Geometry: final body of the model. Coordinates: model frame, mm. Face numbers are marked on the shaded views. A direction names the side the tool comes from. Give positions to 0.01 mm unless a question says otherwise; leave off trailing zeros. Order: outer loops, then holes, each group sorted by start corner. A loop starts at its lowest first (then second) coordinate and runs counter-clockwise, first axis right, second up. Notation, with made-up numbers: (31, 44.5) -> (81, 44.5) arc R32 ccw to (81, 72.5) -> close; hole circle Ø11 at (47.25, 27.5). An arc over 180 degrees is marked (long way). One line per item, written item: value. Start each with the question number.
```python
from build123d import *

# Parameters (mm, degrees)
F0_W     = 37
F0_H     = 37
F0_W_2   = 28
F0_H_2   = 30.4
F1_DEPTH = 4.5
F2_W     = 35
F2_H     = 33
F3_DEPTH = 2
F4_R     = 1.75
F5_DEPTH = 4
F6_DEPTH = 4
F7_R     = 1


with BuildPart() as f1:
    # F0 (on Top) → F1 (new body)
    with BuildSketch(Plane.XY):
        with Locations((-7.463294, -0.689729)):
            Rectangle(F0_W, F0_H)
        with Locations((-6.963294, -0.689729)):
            Rectangle(F0_W_2, F0_H_2, mode=Mode.SUBTRACT)
    extrude(amount=F1_DEPTH)

    # F2 (on face) → F3 (cut)
    with BuildSketch(Plane.XY.offset(4.5)):
        with Locations((-8.463294, -0.689729)):
            Rectangle(F2_W, F2_H)
    extrude(amount=-F3_DEPTH, mode=Mode.SUBTRACT)

    # F4 (on Top) → F5 (join)
    with BuildSketch(Plane.XY):
        with BuildLine():
            Line((-13.963294, 17.810271), (-13.963294, 22.810271))
            ThreePointArc((-13.963294, 22.810271), (-18.963294, 27.810271), (-23.963294, 22.810271))
            Line((-23.963294, 22.810271), (-23.963294, 17.810271))
            Line((-23.963294, 17.810271), (-13.963294, 17.810271))
        make_face()
        with Locations((-18.963294, 22.810271)):
            Circle(F4_R, mode=Mode.SUBTRACT)
        with BuildLine():
            Line((-23.963294, -19.189729), (-23.963294, -24.189729))
            ThreePointArc((-23.963294, -24.189729), (-18.963294, -29.189729), (-13.963294, -24.189729))
            Line((-13.963294, -24.189729), (-13.963294, -19.189729))
            Line((-13.963294, -19.189729), (-23.963294, -19.189729))
        make_face()
        with Locations((-18.963294, -24.189729)):
            Circle(F4_R, mode=Mode.SUBTRACT)
    extrude(amount=F5_DEPTH)

    # F4 (on Top) → F6 (join)
    with BuildSketch(Plane.XY):
        with BuildLine():
            Line((-13.963294, 17.810271), (-13.963294, 22.810271))
            ThreePointArc((-13.963294, 22.810271), (-18.963294, 27.810271), (-23.963294, 22.810271))
            Line((-23.963294, 22.810271), (-23.963294, 17.810271))
            Line((-23.963294, 17.810271), (-13.963294, 17.810271))
        make_face()
        with Locations((-18.963294, 22.810271)):
            Circle(F4_R, mode=Mode.SUBTRACT)
        with BuildLine():
            Line((-23.963294, -19.189729), (-23.963294, -24.189729))
            ThreePointArc((-23.963294, -24.189729), (-18.963294, -29.189729), (-13.963294, -24.189729))
            Line((-13.963294, -24.189729), (-13.963294, -19.189729))
            Line((-13.963294, -19.189729), (-23.963294, -19.189729))
        make_face()
        with Locations((-18.963294, -24.189729)):
            Circle(F4_R, mode=Mode.SUBTRACT)
    extrude(amount=F6_DEPTH)

    # F7
    f7_edges = [f1.edges().sort_by_distance(p)[0] for p in [
        (7.036706, 14.510271, 1.25),
        (-20.963294, 14.510271, 1.25),
        (-20.963294, -15.889729, 1.25),
        (7.036706, -15.889729, 1.25),
        (-25.963294, -19.189729, 2.25),
        (-25.963294, 17.810271, 2.25),
    ]]
    fillet(f7_edges, radius=F7_R)


solid = f1.part
```
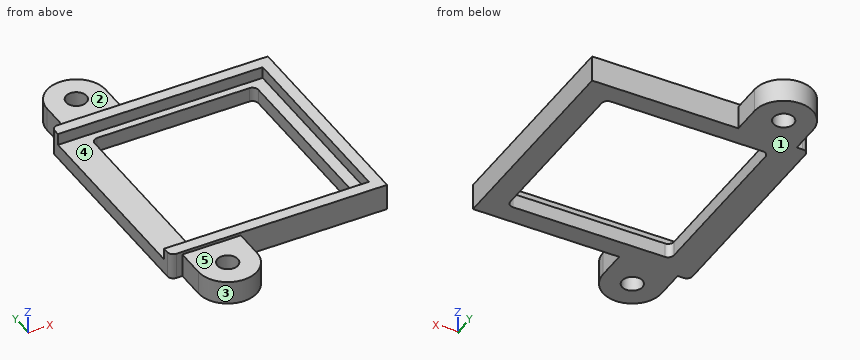
1. Pin query (flat end, axial travel): P1, Ø1.2, axis at y = -22, z = 2, coming from the +X side; P2, Ø0.8, axis at x = -2, z = 1.5, coming from the +Y side; P3, Ø1, axis at x = -2.5, z = 3.5, coming from the -Y side. Return the tip coordinate at first contact, or that it passes through.
2. Cut plane B-B, the plane z = 0.6. Return loops of the section in (x, y).
3. Cut plane D-D, the plane z = 3.4. Return loops of the section in (x, y).
4. Draft query along Y for the marked faces 3, 4 and 5. Return one class per face: pulls with the +Y half, pulls with the -Y half, needs draft (parallel to the pull), parting line crosses it, or undercut.
5. Access query for the marked faces 1 and 2. Directions: +Z, -Z, +X, -X, +Y, -Y. A direction counts if a zero-diameter tool reaches every point of the face in a straight line with its end or side. Return the directions, or none.
6. Cut plane C-C, the plane y = 1. Return loops of the section in (x, z).
7. Cut plane A-A, the plane x = 3. Return loops of the section in (y, z).
8. Material intervals for L1, parallel to Y at x = -9.5, z = 1.45; L2, parallel to Y at x = -9, z = 4.3; L3, parallel to X at y = 3, z = 2.3, sorted ascending. Write a range as [from, to].
Answers follow:
1. P1: stops at x = -13.96
1. P2: stops at y = 17.81
1. P3: stops at y = -19.19
2. outline: (-25.96, -18.19) arc R1 ccw to (-24.96, -19.19) -> (-23.96, -19.19) -> (-23.96, -24.19) arc R5 ccw to (-13.96, -24.19) -> (-13.96, -19.19) -> (11.04, -19.19) -> (11.04, 17.81) -> (-13.96, 17.81) -> (-13.96, 22.81) arc R5 ccw to (-23.96, 22.81) -> (-23.96, 17.81) -> (-24.96, 17.81) arc R1 ccw to (-25.96, 16.81) -> close; hole (-20.96, -14.89) arc R1 ccw to (-19.96, -15.89) -> (6.04, -15.89) arc R1 ccw to (7.04, -14.89) -> (7.04, 13.51) arc R1 ccw to (6.04, 14.51) -> (-19.96, 14.51) arc R1 ccw to (-20.96, 13.51) -> close; hole circle Ø3.5 at (-18.96, -24.19); hole circle Ø3.5 at (-18.96, 22.81)
3. outline: (-25.96, -18.19) arc R1 ccw to (-24.96, -19.19) -> (-23.96, -19.19) -> (-23.96, -24.19) arc R5 ccw to (-13.96, -24.19) -> (-13.96, -19.19) -> (11.04, -19.19) -> (11.04, 17.81) -> (-13.96, 17.81) -> (-13.96, 22.81) arc R5 ccw to (-23.96, 22.81) -> (-23.96, 17.81) -> (-24.96, 17.81) arc R1 ccw to (-25.96, 16.81) -> (-25.96, 15.81) -> (9.04, 15.81) -> (9.04, -17.19) -> (-25.96, -17.19) -> close; hole circle Ø3.5 at (-18.96, -24.19); hole circle Ø3.5 at (-18.96, 22.81)
4. face 3: pulls with the -Y half
4. face 4: undercut
4. face 5: needs draft
5. face 1: -Z, +X, -X, +Y, -Y
5. face 2: +Z, +X, -X, +Y
6. outline: (-25.96, 0) -> (-20.96, 0) -> (-20.96, 2.5) -> (-25.96, 2.5) -> close; (7.04, 0) -> (11.04, 0) -> (11.04, 4.5) -> (9.04, 4.5) -> (9.04, 2.5) -> (7.04, 2.5) -> close
7. outline: (-19.19, 0) -> (-15.89, 0) -> (-15.89, 2.5) -> (-17.19, 2.5) -> (-17.19, 4.5) -> (-19.19, 4.5) -> close; (14.51, 0) -> (17.81, 0) -> (17.81, 4.5) -> (15.81, 4.5) -> (15.81, 2.5) -> (14.51, 2.5) -> close
8. L1: y = [-19.19, -15.89], [14.51, 17.81]
8. L2: y = [-19.19, -17.19], [15.81, 17.81]
8. L3: x = [-25.96, -20.96], [7.04, 11.04]
